from build123d import *

# Parameters (mm, degrees)
F0_W         = 22.5927522406
F0_H         = 49.5025906712
F1_DEPTH     = 10.16
F2_DEPTH     = 3.81
F3_W         = 11.2244246993
F3_H         = 99.0051813424
F4_DEPTH     = 25.4
F6_DEPTH     = 10.16
F7_R         = 2.54
F8_W         = 33.9610797819
F8_H         = 38.1342638284
F8_H_2       = 37.1269418392
F9_DEPTH     = 5.842
F10_R        = 2.54
F11_W        = 99.0051813424
F11_H        = 67.9221570026
F11_W_2      = 75.9807229042
F11_H_2      = 8.63417238
F12_DEPTH    = 10.414
F13_W        = 19.139082171
F13_H        = 29.1566260799
F13_W_2      = 6.5123029053
F13_H_2      = 0.8140355349
F13_W_3      = 18.2694643736
F13_W_4      = 7.5298482552
F13_W_5      = 18.2365168585
F13_W_6      = 7.1228295565
F13_W_7      = 18.1018151343
F13_W_8      = 7.1228314191
F14_DEPTH    = 0.254
F15_DEPTH    = 1.524
F16_DEPTH    = 60.96
F17_W        = 8.1115535974
F17_H        = 76.3251371682
F17_W_2      = 2.3215521545
F18_DEPTH    = 55.88
F19_R        = 1.8396307345
F20_T4_DEPTH = 85.1788765768
F21_W        = 35.6879150495
F21_H        = 12.0312273502
F22_DEPTH    = 5.842
F23_R        = 2.54
F24_W        = 76.3251371682
F24_H        = 21.320472064
F25_DEPTH    = 25.4


# Not quite as in the source:
# - a fillet or chamfer that OpenCascade refuses, or shapes differently, is made with other operations: its cross-section is extruded or revolved along the edge and cut away or added
# - a feature names something its author has since deleted; it is built from what else it names


with BuildPart() as f1:
    # F0 (on Top) → F1 (new body)
    with BuildSketch(Plane.XY):
        with BuildLine():
            Line((-35.3594812499, 51.6611337662), (-36.6952344775, 51.6611337662))
            Line((-36.6952344775, 51.6611337662), (-36.6952344775, 50.3253805386))
            ThreePointArc((-36.6952344775, 50.3253805386), (-36.1400711383, 51.105970427), (-35.3594812499, 51.6611337662))
        make_face()
        with BuildLine():
            ThreePointArc((-32.8504798068, 51.6611337662), (-34.1049805284, 51.9489325583), (-35.3594812499, 51.6611337662))
            Line((-35.3594812499, 51.6611337662), (-32.8504798068, 51.6611337662))
        make_face()
        with BuildLine():
            Line((-32.8504798068, 51.6611337662), (-35.3594812499, 51.6611337662))
            ThreePointArc((-35.3594812499, 51.6611337662), (-36.1400711383, 51.105970427), (-36.6952344775, 50.3253805386))
            Line((-36.6952344775, 50.3253805386), (-36.6952344775, 47.8163790954))
            ThreePointArc((-36.6952344775, 47.8163790954), (-33.4614356183, 46.2656993361), (-31.2269277871, 49.070879817))
            ThreePointArc((-31.2269277871, 49.070879817), (-31.6663634179, 50.5993869876), (-32.8504798068, 51.6611337662))
        make_face()
        with BuildLine():
            Line((-36.6952344775, 47.8163790954), (-36.6952344775, 50.3253805386))
            ThreePointArc((-36.6952344775, 50.3253805386), (-36.9830332696, 49.070879817), (-36.6952344775, 47.8163790954))
        make_face()
        with BuildLine():
            Line((-14.1024822369, 51.6611337662), (-32.8504798068, 51.6611337662))
            ThreePointArc((-32.8504798068, 51.6611337662), (-31.6663634179, 50.5993869876), (-31.2269277871, 49.070879817))
            ThreePointArc((-31.2269277871, 49.070879817), (-33.4614356183, 46.2656993361), (-36.6952344775, 47.8163790954))
            Line((-36.6952344775, 47.8163790954), (-36.6952344775, 2.158543095))
            Line((-36.6952344775, 2.158543095), (-14.1024822369, 2.158543095))
            Line((-14.1024822369, 2.158543095), (-14.1024822369, 51.6611337662))
        make_face()
        with Locations((-2.8061061166, 26.9098384306)):
            Rectangle(F0_W, F0_H)
        with BuildLine():
            Line((-14.1024822369, 2.158543095), (-36.6952344775, 2.158543095))
            Line((-36.6952344775, 2.158543095), (-36.6952344775, -43.4992929054))
            ThreePointArc((-36.6952344775, -43.4992929054), (-33.4614356183, -41.9486131461), (-31.2269277871, -44.753793627))
            ThreePointArc((-31.2269277871, -44.753793627), (-31.6663634179, -46.2823007976), (-32.8504798068, -47.3440475762))
            Line((-32.8504798068, -47.3440475762), (-14.1024822369, -47.3440475762))
            Line((-14.1024822369, -47.3440475762), (-14.1024822369, 2.158543095))
        make_face()
        with Locations((-2.8061061166, -22.5927522406)):
            Rectangle(F0_W, F0_H)
        with BuildLine():
            ThreePointArc((-31.2269277871, -44.753793627), (-33.4614356183, -41.9486131461), (-36.6952344775, -43.4992929054))
            Line((-36.6952344775, -43.4992929054), (-36.6952344775, -46.0082943486))
            ThreePointArc((-36.6952344775, -46.0082943486), (-36.1400711383, -46.788884237), (-35.3594812499, -47.3440475762))
            Line((-35.3594812499, -47.3440475762), (-32.8504798068, -47.3440475762))
            ThreePointArc((-32.8504798068, -47.3440475762), (-31.6663634179, -46.2823007976), (-31.2269277871, -44.753793627))
        make_face()
        with BuildLine():
            Line((-36.6952344775, -46.0082943486), (-36.6952344775, -43.4992929054))
            ThreePointArc((-36.6952344775, -43.4992929054), (-36.9830332696, -44.753793627), (-36.6952344775, -46.0082943486))
        make_face()
        with BuildLine():
            ThreePointArc((-35.3594812499, -47.3440475762), (-36.1400711383, -46.788884237), (-36.6952344775, -46.0082943486))
            Line((-36.6952344775, -46.0082943486), (-36.6952344775, -47.3440475762))
            Line((-36.6952344775, -47.3440475762), (-35.3594812499, -47.3440475762))
        make_face()
        with BuildLine():
            ThreePointArc((-35.3594812499, -47.3440475762), (-34.1049805284, -47.6318463683), (-32.8504798068, -47.3440475762))
            Line((-32.8504798068, -47.3440475762), (-35.3594812499, -47.3440475762))
        make_face()
    extrude(amount=F1_DEPTH)

    # F0 (on Top) → F2 (join)
    with BuildSketch(Plane.XY):
        with BuildLine():
            Line((-32.8504798068, 51.6611337662), (-35.3594812499, 51.6611337662))
            ThreePointArc((-35.3594812499, 51.6611337662), (-36.1400711383, 51.105970427), (-36.6952344775, 50.3253805386))
            Line((-36.6952344775, 50.3253805386), (-36.6952344775, 47.8163790954))
            ThreePointArc((-36.6952344775, 47.8163790954), (-33.4614356183, 46.2656993361), (-31.2269277871, 49.070879817))
            ThreePointArc((-31.2269277871, 49.070879817), (-31.6663634179, 50.5993869876), (-32.8504798068, 51.6611337662))
        make_face()
        with BuildLine():
            ThreePointArc((-31.2269277871, -44.753793627), (-33.4614356183, -41.9486131461), (-36.6952344775, -43.4992929054))
            Line((-36.6952344775, -43.4992929054), (-36.6952344775, -46.0082943486))
            ThreePointArc((-36.6952344775, -46.0082943486), (-36.1400711383, -46.788884237), (-35.3594812499, -47.3440475762))
            Line((-35.3594812499, -47.3440475762), (-32.8504798068, -47.3440475762))
            ThreePointArc((-32.8504798068, -47.3440475762), (-31.6663634179, -46.2823007976), (-31.2269277871, -44.753793627))
        make_face()
    extrude(amount=-F2_DEPTH)

    # F3 (on face) → F4 (join)
    with BuildSketch(Plane.XY.offset(10.16)):
        with Locations((2.878057654, 2.158543095)):
            Rectangle(F3_W, F3_H)
    extrude(amount=F4_DEPTH)

    # F5 (on face) → F6 (join)
    with BuildSketch(Plane.XY.offset(10.16)):
        Polygon((-2.7341546956, 40.4367111623), (-2.7341546956, 51.6611337662), (-32.8504798068, 51.6611337662), (-35.3594812499, 51.6611337662), (-36.6952344775, 51.6611337662), (-36.6952344775, 50.3253805386), (-36.6952344775, 47.8163790954), (-36.6952344775, 40.4367111623), align=None)
        Polygon((-2.7341546956, -47.3440475762), (-2.7341546956, -35.8318164945), (-36.6952344775, -35.8318164945), (-36.6952344775, -43.4992929054), (-36.6952344775, -46.0082943486), (-36.6952344775, -47.3440475762), (-35.3594812499, -47.3440475762), (-32.8504798068, -47.3440475762), align=None)
    extrude(amount=F6_DEPTH)

    # F7
    f7_edges = [f1.edges().sort_by_distance(p)[0] for p in [
        (-2.734155, 2.158543, 35.56),
        (-19.714695, -35.831816, 20.32),
        (-19.714695, -47.344048, 20.32),
        (-19.714695, 51.661134, 20.32),
        (-19.714695, 40.436711, 20.32),
    ]]
    fillet(f7_edges, radius=F7_R)

    # F8 (on face) → F9 (join)
    with BuildSketch(Plane.XY.offset(10.16)):
        with Locations((-19.7146945866, 21.3695792481)):
            Rectangle(F8_W, F8_H)
        with Locations((-19.7146945866, -17.2683455748)):
            Rectangle(F8_W, F8_H_2)
    extrude(amount=F9_DEPTH)

    # F10
    f10_edges = [f1.edges().sort_by_distance(p)[0] for p in [
        (-19.714695, 1.295125, 16.002),
        (-19.714695, 2.302447, 16.002),
        (-36.695234, -17.268346, 16.002),
        (-36.695234, 21.369579, 16.002),
    ]]
    fillet(f10_edges, radius=F10_R)

    # F11 (on face) → F12 (join)
    with BuildSketch(Plane.YZ.offset(8.4902700037)):
        with Locations((2.158543095, 30.0757006044)):
            Rectangle(F11_W, F11_H)
        with Locations((2.3897327483, 12.2317448258)):
            Rectangle(F11_W_2, F11_H_2, mode=Mode.SUBTRACT)
    extrude(amount=-F12_DEPTH)

    # F13 (on face) → F14 (join)
    with BuildSketch(Plane(origin=(-1.9237299963, 0, 0), x_dir=(0, -1, 0), z_dir=(-1, 0, 0))):
        with Locations((-30.8671663515, 49.4584660657)):
            Rectangle(F13_W, F13_H)
        with Locations((-30.3225759417, 61.080571264)):
            Rectangle(F13_W_2, F13_H_2, mode=Mode.SUBTRACT)
        with Locations((-11.2932752818, 49.4584660657)):
            Rectangle(F13_W_3, F13_H)
        with Locations((-11.4979553036, 61.080571264)):
            Rectangle(F13_W_4, F13_H_2, mode=Mode.SUBTRACT)
        with Locations((7.7183801332, 49.4584660657)):
            Rectangle(F13_W_5, F13_H)
        with Locations((7.9371919855, 61.080571264)):
            Rectangle(F13_W_6, F13_H_2, mode=Mode.SUBTRACT)
        with Locations((26.7809126526, 49.4584660657)):
            Rectangle(F13_W_7, F13_H)
        with Locations((27.0670773461, 61.080571264)):
            Rectangle(F13_W_8, F13_H_2, mode=Mode.SUBTRACT)
    extrude(amount=F14_DEPTH)

    # F13 (on face) → F15 (join)
    with BuildSketch(Plane(origin=(-1.9237299963, 0, 0), x_dir=(0, -1, 0), z_dir=(-1, 0, 0))):
        with Locations((27.0670773461, 61.080571264)):
            Rectangle(F13_W_8, F13_H_2)
        with Locations((7.9371919855, 61.080571264)):
            Rectangle(F13_W_6, F13_H_2)
        with Locations((-11.4979553036, 61.080571264)):
            Rectangle(F13_W_4, F13_H_2)
        with Locations((-30.3225759417, 61.080571264)):
            Rectangle(F13_W_2, F13_H_2)
    extrude(amount=F15_DEPTH)

    # F11 (on face) → F16 (join)
    with BuildSketch(Plane.YZ.offset(8.4902700037)):
        with Locations((2.3897327483, 12.2317448258)):
            Rectangle(F11_W_2, F11_H_2)
    extrude(amount=-F16_DEPTH)

    # F17 (on face) → F18 (cut)
    with BuildSketch(Plane.XY.offset(64.0367791057)):
        with Locations((2.1320468024, 2.274138853)):
            Rectangle(F17_W, F17_H)
        with Locations((-3.0845060736, 2.274138853)):
            Rectangle(F17_W_2, F17_H)
    extrude(amount=-F18_DEPTH, mode=Mode.SUBTRACT)

    # F19
    f19_edges = [f1.edges().sort_by_distance(p)[0] for p in [
        (-52.46973, 2.389733, 16.548831),
        (-52.46973, 2.389733, 7.914659),
    ]]
    fillet(f19_edges, radius=F19_R)

    # F20: fillet of radius 1.8396307345 on 1 edges, made by hand


with BuildPart() as f20_tool2:
    # F20_s3 → F20_t4 (new body)
    with BuildSketch(Plane.XZ.offset(-44.9791710367)):
        with BuildLine():
            ThreePointArc((-6.0849128853, 16.5488310158), (-4.7840975181, 16.0100156486), (-4.2452821508, 14.7092002813))
            Line((-4.2452821508, 14.7092002813), (-4.2452821508, 16.5488310158))
            Line((-4.2452821508, 16.5488310158), (-6.0849128853, 16.5488310158))
        make_face()
    extrude(amount=F20_T4_DEPTH)

    split(bisect_by=Plane.XZ.offset(-40.4367111623), keep=Keep.TOP)

    split(bisect_by=Plane.XZ.offset(35.8318164945), keep=Keep.BOTTOM)


with BuildPart() as f1_1:
    add(f1.part)

    # F20_t1: cut F20_tool2
    add(f20_tool2.part, mode=Mode.SUBTRACT)

    # F21 (on face) → F22 (join)
    with BuildSketch(Plane.XY.offset(16.5488310158)):
        with Locations((-28.3488673158, 34.3644805253)):
            Rectangle(F21_W, F21_H)
    extrude(amount=F22_DEPTH)

    # F23
    f23_edges = [f1_1.edges().sort_by_distance(p)[0] for p in [
        (-10.50491, 34.364481, 22.390831),
        (-28.348867, 28.348867, 22.390831),
        (-46.192825, 34.364481, 22.390831),
        (-28.348867, 40.380094, 22.390831),
    ]]
    fillet(f23_edges, radius=F23_R)

    # F24 (on face) → F25 (cut)
    with BuildSketch(Plane(origin=(6.1878236011, 0, 0), x_dir=(0, -1, 0), z_dir=(-1, 0, 0))):
        with Locations((-2.274138853, 46.7570151377)):
            Rectangle(F24_W, F24_H)
    extrude(amount=-F25_DEPTH, mode=Mode.SUBTRACT)


solid = f1_1.part
Part model, mm, in its own coordinate system. A direction names the side the tool comes from. Coordinates: 2 decimals unless noted, no trailing zeros. Loops run counter-clockwise (first coordinate to the right, second up) from the corner with the lowest first, then second, coordinate; pieces in that order, holes last. Notation, with made-up numbers: (-5, 83) - (7, 83) arc R24 ccw to (7, 103) - close; hole circle Ø2 at (67, 77). An arc over 180 degrees is marked (long way). Write each question's results on one line, items separated by ' | '. Start each with the question number.
Q1. Slice it at C-C on x = -25.5. Give the cut face in (y, z), and give its area (3 significant figures).
Q2. Which spindle directions (+Z, -Z, +X, -X, +Y, -Y) get a long thin tool onto all of the face, cutting with end or side? Do faces 5 (the flat face through (-29, 34, 22.391)), 6 (the flat face through (7, 3, 36.097)), 7 (the cylindrical face through (-20, -36.6, 19.6)), 8 (the flat face through (-20, 46, 20.32)). Say none if no direction does.
Q3. Slice it at B-B on z = 48.5. Give the cut face in (x, y), and give its area (3 significant figures).
Q4. Slice it at A-A on y = -18. Give the cut face in (x, z), and give its area (3 significant figures).
Q5. Probe line 1 along Y through (x, z) = (-2, 15.5); line 2 along Z through (x, y) = (-28.5, -6); line 3 along X through (y, z) = (22, 26). List the from-to ranges inside material, lowest first.
Q6. Drop flat-ended pins along their axis: pin 1 Ø0.8 at (x, z) = (-34, -1) entering from -Y; pin 2 Ø4 at (x, z) = (5, 49) entering from +Y; pin 3 Ø3 at (x, y) = (-22, 44.5) entering from +Z. Give the stop position or say it passes through.
Q7. Two-plate mould, pull along X, no slides. Class faces 1 (the cylindrical face through (-34.09, 51.95, 5.01)), 2 (the flat face through (-1.924, 46, 50)), 3 (the flat face through (7, 1, 64.037)), 4 (the flat face through (2, 40.437, 36)): +X half, -X half, draft (parallel to the pull), parting line (faces both ways), or undercut.
Q8. Slice it at D-D on y = 36. Give the cut face in (x, z).
Answer:
1) outline: (-47.34, 0) - (51.66, 0) - (51.66, 17.78) arc R2.54 ccw to (49.12, 20.32) - (42.98, 20.32) arc R2.54 ccw to (40.44, 17.78) - (40.44, 16) - (40.38, 16) - (40.38, 19.85) arc R2.54 ccw to (37.84, 22.39) - (30.89, 22.39) arc R2.54 ccw to (28.35, 19.85) - (28.35, 16.55) - (-35.6, 16.55) - (-35.6, 16) - (-35.83, 16) - (-35.83, 17.78) arc R2.54 ccw to (-38.37, 20.32) - (-44.8, 20.32) arc R2.54 ccw to (-47.34, 17.78) - close | area: 1,790 mm2
2) face 5: +Z, -X, +Y, -Y | face 6: +X, -X | face 7: +Z, -X | face 8: +Z, -X, +Y
3) outline: (-1.92, -47.34) - (8.49, -47.34) - (8.49, -35.89) - (-1.92, -35.89) - close; (-1.92, 40.44) - (8.49, 40.44) - (8.49, 51.66) - (-1.92, 51.66) - close | area: 236 mm2
4) outline: (-52.47, 9.75) arc R1.84 ccw to (-50.63, 7.91) - (-36.7, 7.91) - (-36.7, 0) - (-1.92, 0) - (-1.92, -3.89) - (8.49, -3.89) - (8.49, 36.1) - (6.19, 36.1) - (6.19, 8.16) - (-4.25, 8.16) - (-4.25, 14.71) arc R1.84 ccw to (-6.08, 16.55) - (-50.63, 16.55) arc R1.84 ccw to (-52.47, 14.71) - close; (6.19, 57.42) - (8.49, 57.42) - (8.49, 64.04) - (6.19, 64.04) - close | area: 895 mm2
5) line 1: y = -47.34 to -35.89, 40.44 to 51.66 | line 2: z = 0 to 16.55 | line 3: x = 6.19 to 8.49
6) pin 1: stops at y = -47.34 | pin 2: stops at y = 51.66 | pin 3: stops at z = 20.32
7) face 1: parting line | face 2: -X half | face 3: draft | face 4: undercut
8) outline: (-52.47, 9.75) arc R1.84 ccw to (-50.63, 7.91) - (-36.7, 7.91) - (-36.7, 0) - (-1.92, 0) - (-1.92, -3.89) - (8.49, -3.89) - (8.49, 36.1) - (6.19, 36.1) - (6.19, 8.16) - (-4.25, 8.16) - (-4.25, 14.71) arc R1.84 ccw to (-6.08, 16.55) - (-10.5, 16.55) - (-10.5, 19.85) arc R2.54 ccw to (-13.04, 22.39) - (-43.65, 22.39) arc R2.54 ccw to (-46.19, 19.85) - (-46.19, 16.55) - (-50.63, 16.55) arc R1.84 ccw to (-52.47, 14.71) - close; (6.19, 57.42) - (8.49, 57.42) - (8.49, 64.04) - (6.19, 64.04) - close
